from build123d import *

# Parameters (mm, degrees)
F1_DEPTH = 9
F2_R     = 4.49999


# Not quite as in the source:
# - a fillet or chamfer is up to 0.001 mm smaller than in the source, because OpenCascade refuses the exact size


with BuildPart() as f1:
    # F0 (on Top) → F1 (new body)
    with BuildSketch(Plane.XY):
        with BuildLine():
            ThreePointArc((4.5, -8.9302855497), (8.514693183, -5.2440442409), (10, 0))
            ThreePointArc((10, 0), (-5.2440442409, 8.514693183), (-4.5, -8.9302855497))
            Line((-4.5, -8.9302855497), (-4.5, 0))
            ThreePointArc((-4.5, 0), (0, 4.5), (4.5, 0))
            Line((4.5, 0), (4.5, -8.9302855497))
        make_face()
        with BuildLine():
            Line((-4.5, 0), (-4.5, -8.9302855497))
            ThreePointArc((-4.5, -8.9302855497), (0, -10), (4.5, -8.9302855497))
            Line((4.5, -8.9302855497), (4.5, 0))
            ThreePointArc((4.5, 0), (0, -4.5), (-4.5, 0))
        make_face()
        with BuildLine():
            ThreePointArc((4.5, -8.9302855497), (0, -10), (-4.5, -8.9302855497))
            Line((-4.5, -8.9302855497), (-4.5, -50))
            Line((-4.5, -50), (4.5, -50))
            Line((4.5, -50), (4.5, -8.9302855497))
        make_face()
    extrude(amount=F1_DEPTH)

    # F2 (radius 4.5 in the source; OpenCascade refuses exactly that, so slightly less here)
    f2_edges = [f1.edges().sort_by_distance(p)[0] for p in [
        (-4.5, -29.465143, 9),
        (4.5, -29.465143, 9),
        (4.5, -29.465143, 0),
        (-4.5, -29.465143, 0),
    ]]
    fillet(f2_edges, radius=F2_R)


solid = f1.part
Work out the finished part from the listing and answer in its coordinate system (mm). A direction names the side the tool comes from. Round coordinates to 2 decimals unless told otherwise and drop trailing zeros. Write each loop counter-clockwise with the first axis right and the second up, starting at its lowest first coordinate (ties: lowest second). Pieces come first, ordered by that corner, then holes. Notation, with made-up numbers: (46.5, 62) - (52.5, 62) arc R32 cw to (52.5, 88) - close; hole circle Ø1 at (36.25, -15.75). An arc over 180 degrees is marked (long way). Answer in a Markdown table with one row per item. Add a question column.
1. The mould has two halves that part along Y. Classify faces 5 (the cylindrical face through (4.292, -1.352, 4.437)), 6 (the cylindrical face through (3.217, -29.178, 7.647)), 7 (the flat face through (0, -50, 4)): +Y half, -Y half, draft (parallel to the pull), parting line (faces both ways), or undercut.
2. For faces 1 (the flat face through (-2.3, -4.3, 0)), 2 (the cylindrical face through (3.217, -29.178, 1.353)), 3 (the cylindrical face through (-3.217, -29.753, 1.353)), 4 (the cylindrical face through (-3.217, -29.753, 7.647)), determine the directions among +Z, -Z, +X, -X, +Y, -Y from which every point of the face is accessible in a straight line to the end or side of a thin tool.
3. A cutting plane is placed at D-D, the plane x = -3. Determine the outline of the cut face in (y, z).
4. Given pin 1 (4 mm diameter, centred on y = -5, z = 4.5, fed in from -X); pin 2 (5.5 mm diameter, centred on x = 0, y = 0, fed in from +Z); pin 3 (1.5 mm diameter, centred on x = 2.5, y = -42.5, fed in from -Z), each flat-ended and moving along its own axis, determine where each tip first touches the part or whether it passes through.
5. Find the intervals of material crossed by line 1 along X through (y, z) = (0, 7); line 2 along Y through (x, z) = (0, 5); line 3 along X through (y, z) = (-40, 4.25), in increasing order. Write a range as from..to.
6. A cutting plane is placed at C-C, the plane z = 3. Determine the outline of the cut face in (x, y).
7. A cutting plane is placed at A-A, the plane x = 3.25. Determine the outline of the cut face in (y, z), and give its area (3 significant figures).
Worked out:
| question | item | result |
|---|---|---|
| 1 | face 5 | undercut |
| 1 | face 6 | draft |
| 1 | face 7 | -Y half |
| 2 | face 1 | -Z, +X, -X, +Y, -Y |
| 2 | face 2 | -Z, +X, -Y |
| 2 | face 3 | -Z, -X, -Y |
| 2 | face 4 | +Z, -X, -Y |
| 3 | outline | (-50, 1.15) - (-9.54, 1.15) - (-9.54, 0) - (-3.35, 0) - (-3.35, 9) - (-9.54, 9) - (-9.54, 7.85) - (-50, 7.85) - close; (3.35, 0) - (9.54, 0) - (9.54, 9) - (3.35, 9) - close |
| 4 | pin 1 | x = -9.54 |
| 4 | pin 2 | through |
| 4 | pin 3 | z = 0.35 |
| 5 | line 1 | -10..-4.5, 4.5..10 |
| 5 | line 2 | -50..-4.5, 4.5..10 |
| 5 | line 3 | -4.49..4.49 |
| 6 | outline | (-4.24, -50) - (4.24, -50) - (4.24, -9.06) arc R10 ccw (long way) to (-4.24, -9.06) - close; hole circle Ø9 at (0, 0) |
| 7 | outline | (-50, 1.39) - (-9.46, 1.39) - (-9.46, 0) - (-3.11, 0) - (-3.11, 9) - (-9.46, 9) - (-9.46, 7.61) - (-50, 7.61) - close; (3.11, 0) - (9.46, 0) - (9.46, 9) - (3.11, 9) - close |
| 7 | area | 367 mm^2 |
